For this review, take the finished solid that the model builds, in its own axes (mm). A direction names the side the tool comes from. Coordinates: 2 decimals unless noted, no trailing zeros. Loops run counter-clockwise (first coordinate to the right, second up) from the corner with the lowest first, then second, coordinate; pieces in that order, holes last. Notation, with made-up numbers: M 58,61 L 85,61 A25 cw 85,90 Z; hole C 24,75.25 d10. An arc over 180 degrees is marked long. Put each result on its own line as item: value.
```python
from build123d import *

# Parameters (mm, degrees)
SKETCH1_W           = 9
SKETCH1_H           = 9
BOSS_EXTRUDE1_DEPTH = 3
SKETCH2_W           = 2.95
SKETCH2_H           = 6
BOSS_EXTRUDE2_DEPTH = 6.1
FILLET1_R           = 3
SKETCH3_R           = 0.975
CUT_EXTRUDE1_DEPTH  = 11.1
CUT_EXTRUDE3_DEPTH  = 21.1
BOSS_EXTRUDE3_START = 4
SKETCH5_R           = 3
BOSS_EXTRUDE3_DEPTH = 4
SKETCH8_R           = 1.55
CUT_EXTRUDE4_DEPTH  = 3
CUT_EXTRUDE5_DEPTH  = 0.5
BOSS_EXTRUDE4_START = 4
BOSS_EXTRUDE4_DEPTH = 4
BOSS_EXTRUDE5_DEPTH = 0.5
BOSS_EXTRUDE6_DEPTH = 0.5
SKETCH15_W          = 0.501923789
SKETCH15_H          = 0.5
CUT_EXTRUDE6_DEPTH  = 19.5
SKETCH16_R          = 1.45
CUT_EXTRUDE7_DEPTH  = 19.5
FILLET2_R           = 0.5


with BuildPart() as part:
    # Sketch1 → Boss-Extrude1 (new body)
    with BuildSketch(Plane(origin=(0, 0, 0), x_dir=(1, 0, 0), z_dir=(0, 1, 0))):
        with Locations((4.5, 4.5)):
            Rectangle(SKETCH1_W, SKETCH1_H)
    extrude(amount=BOSS_EXTRUDE1_DEPTH)

    # Sketch2 → Boss-Extrude2 (add)
    with BuildSketch(Plane(origin=(0, 0, -9), x_dir=(-1, 0, 0), z_dir=(0, 0, -1))):
        with Locations((-7.525, 1.5)):
            Rectangle(SKETCH2_W, SKETCH2_H)
        with Locations((-1.475, 1.5)):
            Rectangle(SKETCH2_W, SKETCH2_H)
    extrude(amount=BOSS_EXTRUDE2_DEPTH)

    # Fillet1
    fillet1_edges = [part.edges().sort_by_distance(p)[0] for p in [
        (1.475, 4.5, -15.1),
        (1.475, -1.5, -15.1),
        (7.525, -1.5, -15.1),
        (7.525, 4.5, -15.1),
    ]]
    fillet(fillet1_edges, radius=FILLET1_R - 0.0001)  # a hair under: the kernel refuses the full size

    # Sketch3 → Cut-Extrude1 (cut)
    with BuildSketch(Plane(origin=(9, 0, 0), x_dir=(0, 0, -1), z_dir=(1, 0, 0))):
        with Locations((12.1, 1.5)):
            Circle(SKETCH3_R)
    extrude(amount=-CUT_EXTRUDE1_DEPTH, mode=Mode.SUBTRACT)

    # Sketch6 → Cut-Extrude3 (cut)
    with BuildSketch(Plane.ZY):
        with BuildLine():
            Line((-12.1, 4.5), (-9, 4.5))
            Line((-9, 4.5), (-9, 3))
            Line((-9, 3), (-9.501923789, 3))
            ThreePointArc((-9.501923789, 3), (-10.6, 4.098076211), (-12.1, 4.5))
        make_face()
        with BuildLine():
            Line((-12.1, -1.5), (-9, -1.5))
            Line((-9, -1.5), (-9, 0))
            Line((-9, 0), (-9.501923789, 0))
            ThreePointArc((-9.501923789, 0), (-10.6, -1.098076211), (-12.1, -1.5))
        make_face()
    extrude(amount=-CUT_EXTRUDE3_DEPTH, mode=Mode.SUBTRACT)

    # Sketch5 → Boss-Extrude3 (add)
    with BuildSketch(Plane.ZY.offset(BOSS_EXTRUDE3_START)):
        with Locations((-12.1, 1.5)):
            Circle(SKETCH5_R)
    extrude(amount=-BOSS_EXTRUDE3_DEPTH)

    # Sketch8 → Cut-Extrude4 (cut)
    with BuildSketch(Plane(origin=(0, -1.5, 0), x_dir=(-1, 0, 0), z_dir=(0, -1, 0))):
        with Locations(Location((1.6, 12.1, 0), (0, 0, 90))):
            Circle(SKETCH8_R)
    extrude(amount=-CUT_EXTRUDE4_DEPTH, mode=Mode.SUBTRACT)

    # Sketch9 → Cut-Extrude5 (cut)
    with BuildSketch(Plane.ZY.offset(4)):
        with BuildLine():
            Line((-11.85, 1.5), (-11.85, -0.8))
            ThreePointArc((-11.85, -0.8), (-12.1, -1.05), (-12.35, -0.8))
            Line((-12.35, -0.8), (-12.35, 0.896446609))
            Line((-12.35, 0.896446609), (-13.549568901, -0.303122292))
            ThreePointArc((-13.549568901, -0.303122292), (-13.903122292, -0.303122292), (-13.903122292, 0.050431099))
            Line((-13.903122292, 0.050431099), (-12.703553391, 1.25))
            Line((-12.703553391, 1.25), (-14.4, 1.25))
            ThreePointArc((-14.4, 1.25), (-14.65, 1.5), (-14.4, 1.75))
            Line((-14.4, 1.75), (-12.703553391, 1.75))
            Line((-12.703553391, 1.75), (-13.903122292, 2.949568901))
            ThreePointArc((-13.903122292, 2.949568901), (-13.903122292, 3.303122292), (-13.549568901, 3.303122292))
            Line((-13.549568901, 3.303122292), (-12.35, 2.103553391))
            Line((-12.35, 2.103553391), (-12.35, 3.8))
            ThreePointArc((-12.35, 3.8), (-12.1, 4.05), (-11.85, 3.8))
            Line((-11.85, 3.8), (-11.85, 1.5))
        make_face()
    extrude(amount=-CUT_EXTRUDE5_DEPTH, mode=Mode.SUBTRACT)

    # Sketch10 → Boss-Extrude4 (add)
    with BuildSketch(Plane.ZY.offset(BOSS_EXTRUDE4_START)):
        with BuildLine():
            Line((-9.501923789, 0), (0, 0))
            Line((0, 0), (0, 3))
            Line((0, 3), (-9.501923789, 3))
            ThreePointArc((-9.501923789, 3), (-9.1, 1.5), (-9.501923789, 0))
        make_face()
    extrude(amount=-BOSS_EXTRUDE4_DEPTH)

    # Sketch12 → Boss-Extrude5 (add)
    with BuildSketch(Plane.XZ):
        Polygon((9, 0), (-4, 0), (-4, -9.501923789), (2.95, -9.501923789), (2.95, -9), (6.05, -9), (6.05, -9.501923789), (9, -9.501923789), align=None)
    extrude(amount=BOSS_EXTRUDE5_DEPTH)

    # Sketch13 → Boss-Extrude6 (add)
    with BuildSketch(Plane(origin=(0, 3, 0), x_dir=(1, 0, 0), z_dir=(0, 1, 0))):
        Polygon((2.95, 9.501923789), (-4, 9.501923789), (-4, 0), (9, 0), (9, 9.501923789), (6.05, 9.501923789), (6.05, 9), (2.95, 9), align=None)
    extrude(amount=BOSS_EXTRUDE6_DEPTH)

    # Sketch15 → Cut-Extrude6 (cut)
    with BuildSketch(Plane(origin=(9, 0, 0), x_dir=(0, 0, -1), z_dir=(1, 0, 0))):
        with Locations((9.250961895, 3.25)):
            Rectangle(SKETCH15_W, SKETCH15_H)
        with Locations((9.250961895, -0.25)):
            Rectangle(SKETCH15_W, SKETCH15_H)
    extrude(amount=-CUT_EXTRUDE6_DEPTH, mode=Mode.SUBTRACT)

    # Sketch16 → Cut-Extrude7 (cut)
    with BuildSketch(Plane(origin=(0, 3.5, 0), x_dir=(1, 0, 0), z_dir=(0, 1, 0))):
        with Locations(Location((6, 3, 0), (0, 0, 270))):
            Circle(SKETCH16_R)
        with Locations(Location((-1, 3, 0), (0, 0, 90))):
            Circle(SKETCH16_R)
    extrude(amount=-CUT_EXTRUDE7_DEPTH, mode=Mode.SUBTRACT)

    # Fillet2
    fillet2_edges = [part.edges().sort_by_distance(p)[0] for p in [
        (2.5, 3.5, 0),
        (9, 1.25, 0),
        (2.5, -0.5, 0),
        (-4, 1.5, 0),
        (-4, -0.5, -4.5),
        (-4, 3.5, -4.5),
        (9, 3.5, -4.5),
        (9, -0.5, -4.5),
        (2.5, 3.5, -9),
        (2.5, -0.5, -9),
    ]]
    fillet(fillet2_edges, radius=FILLET2_R - 0.0001)  # a hair under: the kernel refuses the full size


solid = part.part
```
(1) Add section A-A (x = 7). State how many separate pieces and enclosed holes the cut face has, plus the area to 3 significant figures.
Determined:
separate pieces: 2
enclosed holes: 1
area: 53.4 mm^2
(2) For pin 1 (1.6 mm diameter, centred on y = 1.5, z = -12.1, fed in from +X); pin 2 (1 mm diameter, centred on x = -0.5, z = -5.5, fed in from +Y); pin 3 (0.9 mm diameter, centred on x = 4.5, y = 1, fed in from -Z), all flat-tipped, find the tip position at first contact; note any pin that passes through.
Determined:
pin 1: stops at x = 0
pin 2: stops at y = 3.5
pin 3: stops at z = -9
(3) Add section D-D (z = -8.25). Write out the cut boundary in (x, y), plus the area to 3 significant figures.
Determined:
outline: M -4,0 A0.5 ccw -3.5,-0.5 L 8.5,-0.5 A0.5 ccw 9,0 L 9,3 A0.5 ccw 8.5,3.5 L -3.5,3.5 A0.5 ccw -4,3 Z
area: 51.8 mm^2
(4) Draft analysis for pull direction Z (two halves, no side actions). For faces 5 (the flat face through (6.05, 1, -11)), 6 (the flat face through (-3.754, 0.642, -13.312)), 7 (the cylindrical face through (1.496, 1.543, -11.126)), 8 (the cylindrical face through (1.45, -0.64, -14.2)), state which applies: +Z half, -Z half, draft (parallel to the pull), parting line (faces both ways), or undercut.
Determined:
face 5: draft
face 6: undercut
face 7: undercut
face 8: -Z half
(5) Wall thickness on line 1 along X through (y, z) = (1.45, -3); line 2 along X through (y, z) = (3.5, -13.5); line 3 along X through (y, z) = (3.25, -1.75): over which ranges is each line inside the solid? List them lowest first. Write a range as [from, to].
Determined:
line 1: x = [-4, -2.45], [0.45, 4.55], [7.45, 9]
line 2: x = [-4, 2.95], [6.05, 9]
line 3: x = [-3.93, -1.73], [-0.27, 5.27], [6.73, 8.93]
(6) Tool access review of faces 1 (the flat face through (0, 2, -12)), 2 (the flat face through (-2, 1.5, -12)), 3 (the flat face through (4, 1, -9)), 4 (the flat face through (-3.754, 2.341, -13.295)): name each direction out of +Z, -Z, +X, -X, +Y, -Y from which nothing blocks a thin tool from reaching the whole face with its end or side.
Determined:
face 1: +X
face 2: -Y
face 3: -Z, +Y, -Y
face 4: -X
